```python
from build123d import *

# Parameters (mm, degrees)
SKETCH2_W           = 19.05
SKETCH2_H           = 19.05
BOSS_EXTRUDE1_DEPTH = 7.62
SKETCH3_W           = 12.7
SKETCH3_H           = 12.7
CUT_EXTRUDE1_DEPTH  = 25.4


with BuildPart() as part:
    # Sketch1 → Revolve1 (revolve)
    with BuildSketch(Plane.XY):
        Polygon((0, 0), (0, 122.2375), (26.9875, 122.2375), (26.9875, 119.6975), (34.13125, 105.7275), (34.13125, 7.62), (26.9875, 2.54), (26.9875, 0), align=None)
    revolve(axis=Axis((0, 0, 0), (0, 1, 0)))

    # Sketch2 → Boss-Extrude1 (add)
    with BuildSketch(Plane.ZY.offset(34.13125)):
        with Locations((0, 17.145)):
            Rectangle(SKETCH2_W, SKETCH2_H)
    extrude(amount=-BOSS_EXTRUDE1_DEPTH)

    # Sketch3 → Cut-Extrude1 (cut)
    with BuildSketch(Plane.XZ):
        with Locations((6.35, 6.35)):
            Rectangle(SKETCH3_W, SKETCH3_H)
    extrude(amount=-CUT_EXTRUDE1_DEPTH, mode=Mode.SUBTRACT)


solid = part.part
```
Could you check a few things on this model? Use its own coordinates, in mm. A direction names the side the tool comes from. Round coordinates to 2 decimals unless told otherwise and drop trailing zeros. Loops run counter-clockwise (first coordinate to the right, second up) from the corner with the lowest first, then second, coordinate; pieces in that order, holes last.
Q1. On a 3-axis mill with a long thin cutter (end or side, diameter ignored), from which of +Z, -Z, +X, -X, +Y, -Y can I reach the whole of each face in a straight line? I mean faces 1 (the cylindrical face through (-19.89, 120.95, -18.24)), 2 (the flat face through (12.7, 13, 6)), 3 (the flat face through (0, 122.238, 0)). Say none if no direction works.
Q2. I want a section at B-B (y = 113). Write out the boundary of the cut face in (x, z).
Q3. I want a section at A-A (y = 85). Write out the boundary of the cut face in (x, z), and give its area (3 significant figures).
Q4. Please list where these lines run through material, in increasing order: L1, parallel to X at y = 49.5, z = -1; L2, parallel to Z at x = 6, y = 11.5; L3, parallel to Z at x = 0, y = 104.
Q5. Thinking about a two-plate mould opening in Z: for faces 4 (the cylindrical face through (32.555, 55.987, -10.252)), 5 (the flat face through (6, 13, 12.7)), 6 (the flat face through (-34.131, 17, 0)), 7 (the flat face through (0, 13, 6)), which applies, pulls with the +Z half, pulls with the -Z half, needs draft (parallel to the pull), parting line crosses it, or undercut?
Q6. For P1, Ø10, axis at x = -5.5, z = 14.5, coming from the -Y side; P2, Ø14, axis at y = 14.5, z = 8, coming from the +X side; P3, Ø4, axis at x = 20.5, y = 36.5, coming from the +Z side; P4, Ø5, axis at x = 15, y = 62.5, coming from the -Z side, each with a flat end and sliding along its axis, tell me the tip position at first contact or that it passes through.
Answer below:
1. face 1: +Y
1. face 2: -Y
1. face 3: +Z, -Z, +X, -X, +Y
2. outline: circle Ø60.82 at (0, 0)
3. outline: circle Ø68.26 at (0, 0)
3. area: 3,660 mm2
4. L1: x = -34.12 to 34.12
4. L2: z = -33.6 to 0, 12.7 to 33.6
4. L3: z = -34.13 to 34.13
5. face 4: parting line crosses it
5. face 5: undercut
5. face 6: needs draft
5. face 7: undercut
6. P1: stops at y = 0
6. P2: stops at x = 34.12
6. P3: stops at z = 28.68
6. P4: stops at z = -31.76
